```python
from build123d import *

# Parameters (mm, degrees)
F0_W     = 12
F0_H     = 12
F0_R     = 4
F1_DEPTH = 15
F2_W     = 25
F2_H     = 12
F3_DEPTH = 5
F4_W     = 3
F4_H     = 8
F5_DEPTH = 5


with BuildPart() as f1:
    # F0 (on Top) → F1 (new body)
    with BuildSketch(Plane.XY):
        Rectangle(F0_W, F0_H)
        Circle(F0_R, mode=Mode.SUBTRACT)
    extrude(amount=F1_DEPTH)

    # F2 (on face) → F3 (join)
    with BuildSketch(Plane(origin=(0, 0, 0), x_dir=(1, 0, 0), z_dir=(0, 0, -1))):
        Rectangle(F2_W, F2_H)
    extrude(amount=F3_DEPTH)

    # F4 (on face) → F5 (cut)
    with BuildSketch(Plane.XY):
        with Locations((-9.25, 0)):
            Rectangle(F4_W, F4_H)
        with Locations((9.25, 0)):
            Rectangle(F4_W, F4_H)
    extrude(amount=-F5_DEPTH, mode=Mode.SUBTRACT)


solid = f1.part
```
Verification items for the finished model (mm, model axes). A direction names the side the tool comes from. Give positions to 0.01 mm unless a question says otherwise; leave off trailing zeros. Loops run counter-clockwise (first coordinate to the right, second up) from the corner with the lowest first, then second, coordinate; pieces in that order, holes last.
1. Section check A-A, the plane y = 0. Enter the section's corners in (x, z), then the cut area to 3 significant figures.
2. Section check C-C, the plane z = 13.5. Enter the section's corners in (x, y).
3. Section check D-D, the plane x = 0. Enter the section's corners in (y, z).
4. Set-up check for faces 1 (the flat face through (6, 0, 7)), 2 (the cylindrical face through (-0.867, -3.905, 7.395)), 3 (the flat face through (-7, 0, 0)), 4 (the flat face through (-7.75, 0, -2)): record each of +Z, -Z, +X, -X, +Y, -Y from which the full face is reachable in a straight line by a thin tool's end or side.
5. Go/stop test with flat-tipped pins: pin 1 Ø1 at (y, z) = (1.5, 11.5) entering from +X; pin 2 Ø2.5 at (x, y) = (1, 1.5) entering from +Z; pin 3 Ø6 at (y, z) = (0.5, 8) entering from -X. Record where each tip stops, or that it passes through.
6. Section check B-B, the plane x = 9.25. Enter the section's corners in (y, z).
7. Mould release check, pull along X, two halves, no side actions. Record for faces 5 (the flat face through (-1.4, 4.1, 15)), 6 (the flat face through (-9, 4, -2)), 7 (the flat face through (12.5, 0, -2)): released by +X, released by -X, zero draft, split by the parting line, or undercut.
8. Thickness scan on line 1 (X direction, y = 2, z = -1.75); line 2 (Z direction, x = 1, y = 3.25); line 3 (X direction, y = -5, z = 11). Record the ranges inside material, lowest first.
Geometry says:
1. outline: (-12.5, -5) - (-10.75, -5) - (-10.75, 0) - (-12.5, 0) - close; (-7.75, -5) - (7.75, -5) - (7.75, 0) - (6, 0) - (6, 15) - (4, 15) - (4, 0) - (-4, 0) - (-4, 15) - (-6, 15) - (-6, 0) - (-7.75, 0) - close; (10.75, -5) - (12.5, -5) - (12.5, 0) - (10.75, 0) - close
1. area: 155 mm2
2. outline: (-6, -6) - (6, -6) - (6, 6) - (-6, 6) - close; hole circle Ø8 at (0, 0)
3. outline: (-6, -5) - (6, -5) - (6, 15) - (4, 15) - (4, 0) - (-4, 0) - (-4, 15) - (-6, 15) - close
4. face 1: +Z, +X, +Y, -Y
4. face 2: +Z
4. face 3: +Z, -X, +Y, -Y
4. face 4: +Z, -Z
5. pin 1: stops at x = 6
5. pin 2: stops at z = 0
5. pin 3: stops at x = -6
6. outline: (-6, -5) - (-4, -5) - (-4, 0) - (-6, 0) - close; (4, -5) - (6, -5) - (6, 0) - (4, 0) - close
7. face 5: zero draft
7. face 6: undercut
7. face 7: released by +X
8. line 1: x = -12.5 to -10.75, -7.75 to 7.75, 10.75 to 12.5
8. line 2: z = -5 to 0
8. line 3: x = -6 to 6
